Design review of the part built by this model. Coordinates are the model's own, in mm. A direction names the side the tool comes from. Coordinates: 2 decimals unless noted, no trailing zeros. Write each loop counter-clockwise with the first axis right and the second up, starting at its lowest first coordinate (ties: lowest second). Pieces come first, ordered by that corner, then holes. Notation, with made-up numbers: (-35.5, 75) -> (-24.5, 75) arc R26 cw to (-24.5, 105) -> close; hole circle Ø3 at (48.25, -12.75). An arc over 180 degrees is marked (long way). Return JSON: item names as keys, results as strings. Group by question number.
from build123d import *

# Parameters (mm, degrees)
ESQUISSE2_W             = 65
ESQUISSE2_H             = 14
BOSS_EXTRU_1_DEPTH      = 4
ESQUISSE3_R             = 5.5
ENL_V_MAT_EXTRU_1_DEPTH = 2
ESQUISSE4_R             = 3.5
ENL_V_MAT_EXTRU_2_DEPTH = 38.080787511
BOSS_EXTRU_3_DEPTH      = 14
ESQUISSE7_R             = 12.5
ENL_V_MAT_EXTRU_4_DEPTH = 39.788005272
ESQUISSE8_R             = 1.5
ENL_V_MAT_EXTRU_5_DEPTH = 38.362880007
CHANFREIN1_SIZE         = 1
CHANFREIN2_SIZE         = 4


with BuildPart() as part:
    # Esquisse2 → Boss.-Extru.1 (new body)
    with BuildSketch(Plane(origin=(0, 0, 0), x_dir=(1, 0, 0), z_dir=(0, 1, 0))):
        with Locations((-3.326098768, -2.352831094)):
            Rectangle(ESQUISSE2_W, ESQUISSE2_H)
    extrude(amount=-BOSS_EXTRU_1_DEPTH)

    # Esquisse3 → Enlèv. mat.-Extru.1 (cut)
    with BuildSketch(Plane.XZ.offset(4)):
        with Locations(Location((-28.826098768, 2.352831094, 0), (0, 0, 270))):
            Circle(ESQUISSE3_R)
        with Locations(Location((22.173901232, 2.352831094, 0), (0, 0, 270))):
            Circle(ESQUISSE3_R)
    extrude(amount=-ENL_V_MAT_EXTRU_1_DEPTH, mode=Mode.SUBTRACT)

    # Esquisse4 → Enlèv. mat.-Extru.2 (cut, through all)
    with BuildSketch(Plane.XZ.offset(2)):
        with Locations(Location((-28.826098768, 2.352831094, 0), (0, 0, 270))):
            Circle(ESQUISSE4_R)
        with Locations(Location((22.173901232, 2.352831094, 0), (0, 0, 270))):
            Circle(ESQUISSE4_R)
    extrude(amount=-ENL_V_MAT_EXTRU_2_DEPTH, mode=Mode.SUBTRACT)

    # Esquisse5 → Boss.-Extru.3 (add)
    with BuildSketch(Plane(origin=(0, 0, -4.647168906), x_dir=(-1, 0, 0), z_dir=(0, 0, -1))):
        with BuildLine():
            Line((-10.421628317, -4), (17.073825853, -4))
            ThreePointArc((17.073825853, -4), (3.326098768, 5), (-10.421628317, -4))
        make_face()
    extrude(amount=-BOSS_EXTRU_3_DEPTH)

    # Esquisse7 → Enlèv. mat.-Extru.4 (cut, through all)
    with BuildSketch(Plane(origin=(0, 0, -4.647168906), x_dir=(-1, 0, 0), z_dir=(0, 0, -1))):
        with Locations((3.326098768, -10)):
            Circle(ESQUISSE7_R)
    extrude(amount=-ENL_V_MAT_EXTRU_4_DEPTH, mode=Mode.SUBTRACT)

    # Esquisse8 → Enlèv. mat.-Extru.5 (cut, through all)
    with BuildSketch(Plane(origin=(0, 0, 0), x_dir=(1, 0, 0), z_dir=(0, 1, 0))):
        with Locations(Location((-20.326098768, -2.352831094, 0), (0, 0, 270))):
            Circle(ESQUISSE8_R)
        with Locations(Location((13.673901232, -2.352831094, 0), (0, 0, 270))):
            Circle(ESQUISSE8_R)
    extrude(amount=-ENL_V_MAT_EXTRU_5_DEPTH, mode=Mode.SUBTRACT)

    # Chanfrein1
    chanfrein1_edges = [part.edges().sort_by_distance(p)[0] for p in [
        (-3.326098768, 5, 9.352831094),
        (-3.326098768, 5, -4.647168906),
    ]]
    chamfer(chanfrein1_edges, length=CHANFREIN1_SIZE)

    # Chanfrein2
    chanfrein2_edges = [part.edges().sort_by_distance(p)[0] for p in [
        (-35.826098768, -2, -4.647168906),
        (29.173901232, -2, -4.647168906),
        (29.173901232, -2, 9.352831094),
        (-35.826098768, -2, 9.352831094),
    ]]
    chamfer(chanfrein2_edges, length=CHANFREIN2_SIZE)


solid = part.part
Q1. For faces 1 (the flat face through (-30, -2, -1.2)), 2 (the flat face through (27.202, -1.972, 7.325)), list the 3-axis set-ups (+Z, -Z, +X, -X, +Y, -Y) from which the entire face can be reached by the end or side of a thin tool; tool diameter is ignored.
Q2. For P1, Ø3.5, axis at x = -30.5, z = 0.5, coming from the -Y side; P2, Ø2.5, axis at x = -20.33, z = 2.35, coming from the +Y side; P3, Ø4, axis at x = -26.5, z = 2.5, coming from the +Y side; P4, Ø1, axis at x = -9, z = 4, coming from the -Y side, all flat-tipped, find the tip position at first contact; note any pin that passes through.
Q3. We need section C-C on y = -1. Write out the cut boundary in (x, z), plus the area to 3 significant figures.
Q4. Wall thickness on L1, parallel to X at y = -3, z = 3; L2, parallel to X at y = -0.75, z = 4.25; L3, parallel to X at y = -2.5, z = 1: over which ranges is each line inside the solid? List them lowest first.
Q5. We need section B-B on x = 13. Write out the cut boundary in (y, z).
Q6. We need section A-A on z = 4.75. Write out the cut boundary in (x, y), plus the area to 3 significant figures.
Q7. The part is to be moulded in two halves that separate along Z. For faces 3 (the flat face through (-33.854, -1.972, 7.325)), 4 (the cylindrical face through (-25.356, -1.014, 2.808)), 5 (the cylindrical face through (-3.5, 5, 2.3)), say which applies: +Z half, -Z half, draft (parallel to the pull), parting line (faces both ways), or undercut.
Q8. We need section D-D on z = 1.75. State how many separate pieces and enclosed holes the cut face has, plus the area to 3 significant figures.
Findings below:
{
 "1": {"face 1": "-Y", "face 2": "+Z, +X, +Y, -Y"},
 "2": {"P1": "stops at y = -2", "P2": "passes through", "P3": "stops at y = 0", "P4": "stops at y = 0.87"},
 "3": {"outline": "(-35.83, -0.65) -> (-31.83, -4.65) -> (-12, -4.65) -> (-12, 9.35) -> (-31.83, 9.35) -> (-35.83, 5.35) -> close; (5.35, -4.65) -> (25.17, -4.65) -> (29.17, -0.65) -> (29.17, 5.35) -> (25.17, 9.35) -> (5.35, 9.35) -> close; hole circle Ø7 at (-28.83, 2.35); hole circle Ø3 at (-20.33, 2.35); hole circle Ø3 at (13.67, 2.35); hole circle Ø7 at (22.17, 2.35)", "area": "544 mm^2"},
 "4": {"L1": "x = -35.83 to -34.29, -23.36 to -21.68, -18.97 to -13.68, 7.03 to 12.32, 15.03 to 16.71, 27.64 to 29.17", "L2": "x = -35.83 to -31.77, -25.88 to -11.73, 5.08 to 19.23, 25.12 to 29.17", "L3": "x = -35.83 to -34.16, -23.5 to -20.97, -19.68 to -13.33, 6.67 to 13.03, 14.32 to 16.84, 27.5 to 29.17"},
 "5": {"outline": "(-4, -4.65) -> (0, -4.65) -> (0, 1.01) -> (-4, 1.01) -> close; (-4, 3.69) -> (0, 3.69) -> (0, 9.35) -> (-4, 9.35) -> close"},
 "6": {"outline": "(-35.83, -4) -> (-33.78, -4) -> (-33.78, -2) -> (-31.38, -2) -> (-31.38, 0) -> (-35.83, 0) -> close; (-26.28, -2) -> (-23.88, -2) -> (-23.88, -4) -> (-14.29, -4) arc R12.5 cw to (7.64, -4) -> (17.22, -4) -> (17.22, -2) -> (19.62, -2) -> (19.62, 0) -> (7.85, 0) arc R15 ccw to (-14.51, 0) -> (-26.28, 0) -> close; (24.72, -2) -> (27.12, -2) -> (27.12, -4) -> (29.17, -4) -> (29.17, 0) -> (24.72, 0) -> close", "area": "176 mm^2"},
 "7": {"face 3": "+Z half", "face 4": "undercut", "face 5": "draft"},
 "8": {"separate pieces": "5", "enclosed holes": "0", "area": "143 mm^2"}
}
